from build123d import *

# Parameters (mm, degrees)
SKETCH_1_W         = 43
SKETCH_1_H         = 39
TOP_DEPTH          = 1
DHT22_WINDOW_REACH = 31.043
SKETCH_2_W         = 20.5
SKETCH_2_H         = 15.5
EAR_REACH          = 31.043


with BuildPart() as part:
    # 스케치1 → Top (new body)
    with BuildSketch(Plane(origin=(0, 0, 0), x_dir=(1, 0, 0), z_dir=(0, 1, 0))):
        Rectangle(SKETCH_1_W, SKETCH_1_H)
    extrude(amount=TOP_DEPTH)

    # 스케치2 → DHT22_window (cut, up to next)
    with BuildSketch(Plane(origin=(0, 1, 0), x_dir=(1, 0, 0), z_dir=(0, 1, 0)), mode=Mode.PRIVATE) as dht22_window_sk1:
        with Locations((2, -2)):
            Rectangle(SKETCH_2_W, SKETCH_2_H)
    dht22_window_tool1 = extrude(dht22_window_sk1.sketch, amount=-DHT22_WINDOW_REACH, mode=Mode.PRIVATE) & part.part
    add(dht22_window_tool1.solids().sort_by_distance((2, 1, 2))[0], mode=Mode.SUBTRACT)

    # 스케치3 → Ear (cut, up to next)
    with BuildSketch(Plane.XZ, mode=Mode.PRIVATE) as ear_sk1:
        Polygon((-20, -18), (-20, 18), (-7, 18), (-7, 19.5), (-21.5, 19.5), (-21.5, -19.5), (-7, -19.5), (-7, -18), align=None)
    ear_tool1 = extrude(ear_sk1.sketch, amount=-EAR_REACH, mode=Mode.PRIVATE) & part.part
    # 스케치3 → Ear (cut, up to next)
    with BuildSketch(Plane.XZ, mode=Mode.PRIVATE) as ear_sk2:
        Polygon((7, 19.5), (7, 18), (20, 18), (20, -18), (7, -18), (7, -19.5), (21.5, -19.5), (21.5, 19.5), align=None)
    ear_tool2 = extrude(ear_sk2.sketch, amount=-EAR_REACH, mode=Mode.PRIVATE) & part.part
    add(ear_tool1.solids().sort_by_distance((-7.416083, 0, -18.75))[0], mode=Mode.SUBTRACT)
    add(ear_tool2.solids().sort_by_distance((7.416083, 0, 18.75))[0], mode=Mode.SUBTRACT)


solid = part.part
Build history of the part. All positions in model axes, mm. A direction names the side the tool comes from. Round coordinates to 2 decimals unless told otherwise and drop trailing zeros. Loops run counter-clockwise (first coordinate to the right, second up) from the corner with the lowest first, then second, coordinate; pieces in that order, holes last. Notation, with made-up numbers: (-7, 64.5) -> (38, 64.5) arc R23 cw to (38, 80.5) -> close; hole circle Ø5 at (-19, 69.5). An arc over 180 degrees is marked (long way). One line per item, written item: value. Start each with the question number.
Q1. Cut at B-B on x = 9. List the corners of the cut face in (y, z), plus the area to 3 significant figures.
Q2. Cut at C-C on y = 0.5. List the corners of the cut face in (x, z).
Q3. Probe line 1 along X through (y, z) = (0.9, 4.5); line 2 along Z through (x, y) = (3, 0.4); line 3 along Z through (x, y) = (11.5, 0.8). List the from-to ranges inside material, lowest first.
Q4. 3-axis set-ups, long thin cutter, end or side, ignore diameter. For faces 1 (the face through (-7, 0.5, -18.8)), 2 (the face through (13.6, 0.5, -18)), 3 (the face through (13.4, 0.5, 18)), 4 (the face through (1.9, 0.5, -5.75)), 5 (the face through (-13.6, 0.5, 18)): which of +Z, -Z, +X, -X, +Y, -Y reach the whole face in a straight line?
Q5. Two-plate mould, pull along X, no slides. Class faces 6 (the face through (-13.4, 0.5, -18)), 7 (the face through (7, 0.5, -18.7)), 8 (the face through (-8.25, 0.5, 2.1)), 9 (the face through (1.9, 0.5, 9.75)): released by +X, released by -X, zero draft, split by the parting line, or undercut.
Q6. Drop flat-ended pins along their axis: pin 1 Ø0.5 at (x, y) = (-11, 0.5) entering from -Z; pin 2 Ø0.5 at (x, y) = (13.5, 0.5) entering from +Z; pin 3 Ø0.5 at (y, z) = (0.5, -19) entering from -X. Give the stop position or say it passes through.
Q7. Cut at D-D on x = 14.5. List the corners of the cut face in (y, z), plus the area to 3 significant figures.
Q8. Cut at A-A on z = 4. List the corners of the cut face in (x, y).
Computed:
1. outline: (0, -18) -> (1, -18) -> (1, -5.75) -> (0, -5.75) -> close; (0, 9.75) -> (1, 9.75) -> (1, 18) -> (0, 18) -> close
1. area: 20.5 mm²
2. outline: (-20, -18) -> (-7, -18) -> (-7, -19.5) -> (7, -19.5) -> (7, -18) -> (20, -18) -> (20, 18) -> (7, 18) -> (7, 19.5) -> (-7, 19.5) -> (-7, 18) -> (-20, 18) -> close; hole (-8.25, -5.75) -> (12.25, -5.75) -> (12.25, 9.75) -> (-8.25, 9.75) -> close
3. line 1: -20 to -8.25, 12.25 to 20
3. line 2: -19.5 to -5.75, 9.75 to 19.5
3. line 3: -18 to -5.75, 9.75 to 18
4. face 1: -Z, -X, +Y, -Y
4. face 2: -Z, +X, +Y, -Y
4. face 3: +Z, +X, +Y, -Y
4. face 4: +Y, -Y
4. face 5: +Z, -X, +Y, -Y
5. face 6: zero draft
5. face 7: released by +X
5. face 8: undercut
5. face 9: undercut
6. pin 1: z = -18
6. pin 2: z = 18
6. pin 3: x = -7
7. outline: (0, -18) -> (1, -18) -> (1, 18) -> (0, 18) -> close
7. area: 36.0 mm²
8. outline: (-20, 0) -> (-8.25, 0) -> (-8.25, 1) -> (-20, 1) -> close; (12.25, 0) -> (20, 0) -> (20, 1) -> (12.25, 1) -> close
